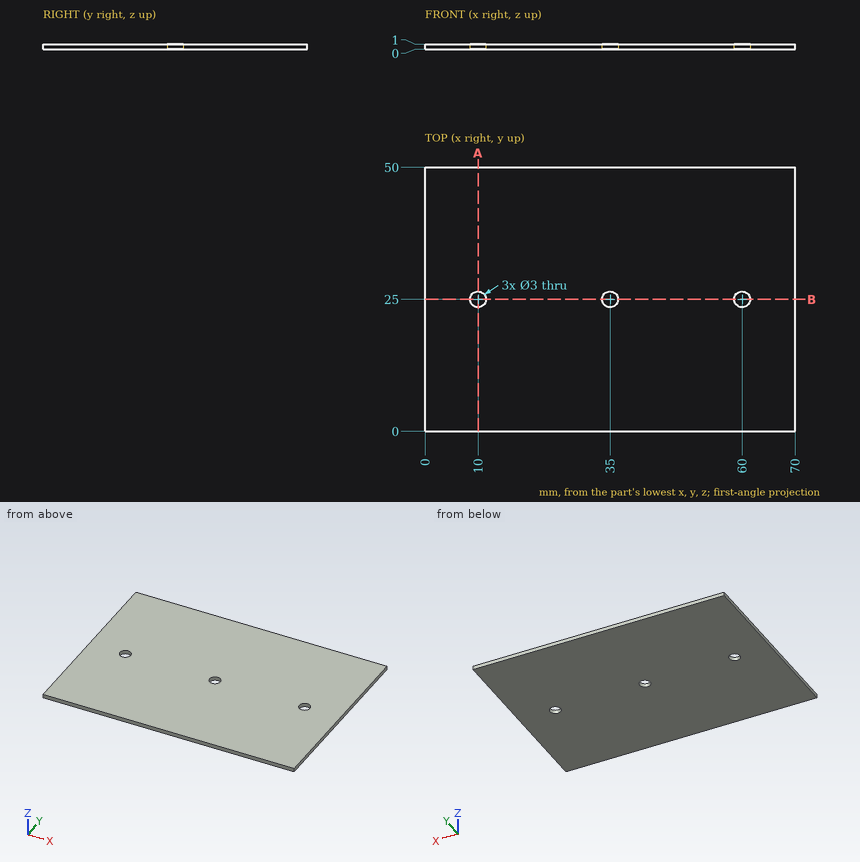
Print and shaded views of the part. All mm, measured from the part's lowest x, y and z. Coordinates: 2 decimals unless noted, no trailing zeros. Write each loop counter-clockwise with the first axis right and the second up, starting at its lowest first coordinate (ties: lowest second). Pieces come first, ordered by that corner, then holes. Notation, with made-up numbers: M -21.75,43.25 L 18.25,43.25 A31 ccw 18.25,68.25 Z; hole C 11.5,53 d7. An arc over 180 degrees is marked long. Return JSON: item names as keys, results as strings.
1. Flat gauge pin, fed straight in: pin 1 Ø1.8 at (x, y) = (10, 25) entering from +Z. Where does the tip first touch, or does it go through?
Determined:
{"pin 1": "through"}
2. Probe L1, parallel to Y at x = 60, z = 0.65; L2, parallel to Y at x = 59, z = 0.25. List the from-to ranges inside material, lowest first.
Determined:
{"L1": "0 to 23.5, 26.5 to 50", "L2": "0 to 23.88, 26.12 to 50"}
3. Saw through at A-A, the plane x = 10. Write the cut outline in (y, z).
Determined:
{"outline": "M 0,0 L 23.5,0 L 23.5,1 L 0,1 Z; M 26.5,0 L 50,0 L 50,1 L 26.5,1 Z"}
4. Saw through at B-B, the plane y = 25. Write the cut outline in (x, z).
Determined:
{"outline": "M 0,0 L 8.5,0 L 8.5,1 L 0,1 Z; M 11.5,0 L 33.5,0 L 33.5,1 L 11.5,1 Z; M 36.5,0 L 58.5,0 L 58.5,1 L 36.5,1 Z; M 61.5,0 L 70,0 L 70,1 L 61.5,1 Z"}
